Source: CAD feature listing. Evaluate the final solid. Frame: model axes, mm. Round coordinates to 2 decimals unless told otherwise and drop trailing zeros. Write each loop counter-clockwise with the first axis right and the second up, starting at its lowest first coordinate (ties: lowest second). Pieces come first, ordered by that corner, then holes.
from build123d import *

# Parameters (mm, degrees)
BOSS_EXTRUDE1_DEPTH          = 4.5
CUT_EXTRUDE1_DEPTH           = 77.442789065
CUT_EXTRUDE1_DEPTH_BACK      = 77.442789065
SKETCH3_R                    = 0.99
SKETCH4_R                    = 5
CUT_EXTRUDE2_DEPTH           = 77.442789065
CUT_EXTRUDE3_DEPTH           = 77.442789065
CUT_EXTRUDE3_DEPTH_BACK      = 77.442789065
SKETCH5_R                    = 1.25
CUT_EXTRUDE4_DEPTH           = 77.442789065
CUT_EXTRUDE4_DEPTH_BACK      = 77.442789065
SKETCH6_R                    = 9.591798866
F_97_0_0059_DIAMETER_HOLE1_D = 0.14986


with BuildPart() as part:
    # Sketch2 → Boss-Extrude1 (new, symmetric)
    with BuildSketch(Plane(origin=(0, 0, 0), x_dir=(1, 0, 0), z_dir=(0, 1, 0))):
        with BuildLine():
            Line((50, -22.5), (-50, -22.5))
            ThreePointArc((-50, -22.5), (-72.5, 0), (-50, 22.5))
            Line((-50, 22.5), (50, 22.5))
            ThreePointArc((50, 22.5), (72.5, 0), (50, -22.5))
        make_face()
    extrude(amount=BOSS_EXTRUDE1_DEPTH, both=True)

    # Sketch3 → Cut-Extrude1 (cut, two sides: drawn at the far end of the back side and taken through both)
    with BuildSketch(Plane(origin=(0, 4.5, 0), x_dir=(1, 0, 0), z_dir=(0, 1, 0)).offset(-CUT_EXTRUDE1_DEPTH_BACK)):
        with Locations(Location((41.95, 0, 0), (0, 0, 270))):
            Circle(SKETCH3_R)
        with Locations(Location((44.307790411, 5.692209589, 0), (0, 0, 270))):
            Circle(SKETCH3_R)
        with Locations(Location((50, 8.05, 0), (0, 0, 270))):
            Circle(SKETCH3_R)
        with Locations(Location((55.692209589, 5.692209589, 0), (0, 0, 270))):
            Circle(SKETCH3_R)
        with Locations(Location((58.05, 0, 0), (0, 0, 270))):
            Circle(SKETCH3_R)
        with Locations(Location((55.692209589, -5.692209589, 0), (0, 0, 270))):
            Circle(SKETCH3_R)
        with Locations(Location((50, -8.05, 0), (0, 0, 270))):
            Circle(SKETCH3_R)
        with Locations(Location((44.307790411, -5.692209589, 0), (0, 0, 270))):
            Circle(SKETCH3_R)
    extrude(amount=CUT_EXTRUDE1_DEPTH + CUT_EXTRUDE1_DEPTH_BACK, mode=Mode.SUBTRACT)

    # Sketch4 → Cut-Extrude2 (cut, through all)
    with BuildSketch(Plane(origin=(0, 4.5, 0), x_dir=(1, 0, 0), z_dir=(0, 1, 0))):
        with Locations(Location((50, 0, 0), (0, 0, 270))):
            Circle(SKETCH4_R)
    extrude(amount=-CUT_EXTRUDE2_DEPTH, mode=Mode.SUBTRACT)

    # Sketch5 → Cut-Extrude3 (cut, two sides: drawn at the far end of the back side and taken through both)
    with BuildSketch(Plane(origin=(0, 4.5, 0), x_dir=(1, 0, 0), z_dir=(0, 1, 0)).offset(-CUT_EXTRUDE3_DEPTH_BACK)):
        with Locations(Location((0, 6, 0), (0, 0, 270))):
            Circle(SKETCH5_R)
        with Locations(Location((0, 0, 0), (0, 0, 270))):
            Circle(SKETCH5_R)
        with Locations(Location((0, -6, 0), (0, 0, 270))):
            Circle(SKETCH5_R)
    extrude(amount=CUT_EXTRUDE3_DEPTH + CUT_EXTRUDE3_DEPTH_BACK, mode=Mode.SUBTRACT)

    # Sketch6 → Cut-Extrude4 (cut, two sides: drawn at the far end of the back side and taken through both)
    with BuildSketch(Plane(origin=(0, 4.5, 0), x_dir=(1, 0, 0), z_dir=(0, 1, 0)).offset(-CUT_EXTRUDE4_DEPTH_BACK)):
        with Locations(Location((-50, 0, 0), (0, 0, 270))):
            Circle(SKETCH6_R)
    extrude(amount=CUT_EXTRUDE4_DEPTH + CUT_EXTRUDE4_DEPTH_BACK, mode=Mode.SUBTRACT)

    # #97 (0.0059) Diameter Hole1 (through all)
    with Locations(Plane(origin=(-21.665942964, -4.5, -0.906896611), x_dir=(0, 0, -1), z_dir=(0, -1, 0))):
        with Locations((0, 0)):
            Hole(F_97_0_0059_DIAMETER_HOLE1_D / 2)


solid = part.part
1) Section query C-C on z = -3. Return the cut outline in (x, y).
Taken from the geometry:
outline: (-72.3, -4.5) - (-59.11, -4.5) - (-59.11, 4.5) - (-72.3, 4.5) - close; (-40.89, -4.5) - (46, -4.5) - (46, 4.5) - (-40.89, 4.5) - close; (54, -4.5) - (72.3, -4.5) - (72.3, 4.5) - (54, 4.5) - close
2) Pull-direction query (X, two-part tool) for faces 1 (the face through (0.05, -0.06, 4.75)), 2 (the face through (72.495, 0.063, -0.495)), 3 (the face through (1, 0, 22.5)), 4 (the face through (-1.22, -0.06, -0.27)); classes: released by +X, released by -X, zero draft, split by the parting line, or undercut.
Taken from the geometry:
face 1: undercut
face 2: released by +X
face 3: zero draft
face 4: undercut
3) Section query A-A on x = 0. Return the cut outline in (y, z).
Taken from the geometry:
outline: (-4.5, -22.5) - (4.5, -22.5) - (4.5, -7.25) - (-4.5, -7.25) - close; (-4.5, -4.75) - (4.5, -4.75) - (4.5, -1.25) - (-4.5, -1.25) - close; (-4.5, 1.25) - (4.5, 1.25) - (4.5, 4.75) - (-4.5, 4.75) - close; (-4.5, 7.25) - (4.5, 7.25) - (4.5, 22.5) - (-4.5, 22.5) - close
4) Section query D-D on y = -2. State how many separate pieces and enclosed holes the cut face has, then the cut area to 3 significant figures.
Taken from the geometry:
separate pieces: 1
enclosed holes: 14
area: 5,680 mm2
5) Contact query for flat-ended pins moving along their axis: P1, Ø3, axis at x = 44.31, z = 5.69, coming from the +Y side; P2, Ø2, axis at y = 2, z = -4.5, coming from the -X side; P3, Ø1, axis at y = -1, z = -11, coming from the +X side; P4, Ø2, axis at y = 0.5, z = -11.5, coming from the -X side. Output: stop coordinate, or through.
Taken from the geometry:
P1: stops at y = 4.5
P2: stops at x = -72.23
P3: stops at x = 69.9
P4: stops at x = -69.9
6) Material intervals for line 1 (X direction, y = 2, z = 0); line 2 (Z direction, x = 0, y = 0.5); line 3 (X direction, y = -4, z = 8), sorted ascending.
Taken from the geometry:
line 1: x = -72.5 to -59.59, -40.41 to -1.25, 1.25 to 40.96, 42.94 to 45, 55 to 57.06, 59.04 to 72.5
line 2: z = -22.5 to -7.25, -4.75 to -1.25, 1.25 to 4.75, 7.25 to 22.5
line 3: x = -71.03 to -55.29, -44.71 to 49.01, 50.99 to 71.03
7) Section query B-B on x = -58. Return the cut outline in (y, z), then the cut area to 3 significant figures.
Taken from the geometry:
outline: (-4.5, -21.03) - (4.5, -21.03) - (4.5, -5.29) - (-4.5, -5.29) - close; (-4.5, 5.29) - (4.5, 5.29) - (4.5, 21.03) - (-4.5, 21.03) - close
area: 283 mm2
